from build123d import *

# Parameters (mm, degrees)
SKETCH1_R           = 2.9
BOSS_EXTRUDE1_DEPTH = 0.25


with BuildPart() as part:
    # Sketch1 → Boss-Extrude1 (new, symmetric)
    with BuildSketch(Plane.XY):
        Polygon((-48.1, 32.1), (48.1, 32.1), (48.1, -32.1), (32.3, -32.1), (32.3, 16.3), (10, 16.3), (10, -32.1), (-10, -32.1), (-10, 16.3), (-32.3, 16.3), (-32.3, -32.1), (-48.1, -32.1), align=None)
        with Locations((40.2, 24.2)):
            Circle(SKETCH1_R, mode=Mode.SUBTRACT)
        with Locations(Location((-40.2, 24.2, 0), (0, 0, 180))):
            Circle(SKETCH1_R, mode=Mode.SUBTRACT)
    extrude(amount=BOSS_EXTRUDE1_DEPTH, both=True)


solid = part.part
For this review, take the finished solid that the model builds, in its own axes (mm). Give positions to 0.01 mm unless a question says otherwise; leave off trailing zeros. Loops run counter-clockwise (first coordinate to the right, second up) from the corner with the lowest first, then second, coordinate; pieces in that order, holes last.
Item 1: Take a section at B-B, the plane x = -40.2. State the section outline as (y, z) points.
Item 2: For line 1 along X through (y, z) = (14.5, -0.1); line 2 along Y through (x, z) = (-40.2, -0.05); line 3 along Y through (x, z) = (-14.5, -0.05), list the stretches that pass through material, from the lowest coordinate up.
Item 3: Draft analysis for pull direction Y (two halves, no side actions). For faces 1 (the flat face through (1, 8, -0.25)), 2 (the cylindrical face through (38.1, 26.2, 0)), state which applies: +Y half, -Y half, draft (parallel to the pull), parting line (faces both ways), or undercut.
Item 4: Insertion check: pin 1 (4.5 mm diameter, centred on x = -40.2, y = 24.2, fed in from +Z) (1 decimal). The pin has a flat end and moves straight along its axis. Give the tip position at first contact, or say it passes through.
Item 5: Take a section at A-A, the plane y = -13. State the section outline as (x, z) points.
Item 6: Take a section at C-C, the plane z = 0.1. State the section outline as (x, y) points, and give its area (3 significant figures).
Item 7: Take a section at D-D, the plane x = 24.5. State the section outline as (y, z) points, and give its area (3 significant figures).
Calculated:
1. outline: (-32.1, -0.25) - (21.3, -0.25) - (21.3, 0.25) - (-32.1, 0.25) - close; (27.1, -0.25) - (32.1, -0.25) - (32.1, 0.25) - (27.1, 0.25) - close
2. line 1: x = -48.1 to -32.3, -10 to 10, 32.3 to 48.1
2. line 2: y = -32.1 to 21.3, 27.1 to 32.1
2. line 3: y = 16.3 to 32.1
3. face 1: draft
3. face 2: undercut
4. pin 1: passes through
5. outline: (-48.1, -0.25) - (-32.3, -0.25) - (-32.3, 0.25) - (-48.1, 0.25) - close; (-10, -0.25) - (10, -0.25) - (10, 0.25) - (-10, 0.25) - close; (32.3, -0.25) - (48.1, -0.25) - (48.1, 0.25) - (32.3, 0.25) - close
6. outline: (-48.1, -32.1) - (-32.3, -32.1) - (-32.3, 16.3) - (-10, 16.3) - (-10, -32.1) - (10, -32.1) - (10, 16.3) - (32.3, 16.3) - (32.3, -32.1) - (48.1, -32.1) - (48.1, 32.1) - (-48.1, 32.1) - close; hole circle Ø5.8 at (-40.2, 24.2); hole circle Ø5.8 at (40.2, 24.2)
6. area: 3,960 mm2
7. outline: (16.3, -0.25) - (32.1, -0.25) - (32.1, 0.25) - (16.3, 0.25) - close
7. area: 7.90 mm2
